```python
from build123d import *

# Parameters (mm, degrees)
F0_R     = 1.5
F0_W     = 8
F0_H     = 3.175
F0_W_2   = 31
F0_H_2   = 9
F0_W_3   = 12
F0_W_4   = 25
F1_DEPTH = 3.175


# Not quite as in the source:
# - a length typed as a fraction of an inch, garbled in the dataset ("3 / 203.2 mm" for 3/8 in), is restored
# - a feature names something its author has since deleted; it is built from what else it names


with BuildPart() as f1:
    # F0 (on Top) → F1 (new body)
    with BuildSketch(Plane.XY):
        Polygon((7.0042573512, 24.8119444549), (-17.9957426488, 24.8119444549), (-17.9957426488, 15.8119444549), (7.0042573512, 15.8119444549), (22.5042573512, 15.8119444549), (38.0042573512, 15.8119444549), (63.0042573512, 15.8119444549), (63.0042573512, 24.8119444549), (38.0042573512, 24.8119444549), align=None)
        with Locations((-13.4957426488, 20.3119444549)):
            Circle(F0_R, mode=Mode.SUBTRACT)
        with Locations((58.5042573512, 20.3119444549)):
            Circle(F0_R, mode=Mode.SUBTRACT)
        Polygon((7.0042573512, 40.6369444549), (7.0042573512, 24.8119444549), (38.0042573512, 24.8119444549), (38.0042573512, 40.6369444549), (30.0042573512, 40.6369444549), (24.0042573512, 40.6369444549), (24.0042573512, 31.3119444549), (25.5042573512, 31.3119444549), (25.5042573512, 29.3119444549), (24.0042573512, 29.3119444549), (24.0042573512, 27.8119444549), (21.0042573512, 27.8119444549), (21.0042573512, 29.3119444549), (19.5042573512, 29.3119444549), (19.5042573512, 31.3119444549), (21.0042573512, 31.3119444549), (21.0042573512, 40.6369444549), (15.0042573512, 40.6369444549), align=None)
        with Locations((11.0042573512, 42.2244444549)):
            Rectangle(F0_W, F0_H)
        Polygon((22.5042573512, 15.8119444549), (7.0042573512, 15.8119444549), (7.0042573512, -12.1880555451), (38.0042573512, -12.1880555451), (38.0042573512, 15.8119444549), align=None)
        with Locations((34.0042573512, 42.2244444549)):
            Rectangle(F0_W, F0_H)
        with Locations((22.5042573512, -16.6880555451)):
            Rectangle(F0_W_2, F0_H_2)
        with Locations((1.0042573512, -16.6880555451)):
            Rectangle(F0_W_3, F0_H_2)
        with Locations((-0.4957426488, -16.6880555451)):
            Circle(F0_R, mode=Mode.SUBTRACT)
        Polygon((38.0042573512, -21.1880555451), (7.0042573512, -21.1880555451), (7.0042573512, -29.0130555451), (15.0042573512, -29.0130555451), (21.0042573512, -29.0130555451), (21.0042573512, -25.6880555451), (19.5042573512, -25.6880555451), (19.5042573512, -23.6880555451), (21.0042573512, -23.6880555451), (21.0042573512, -22.1880555451), (24.0042573512, -22.1880555451), (24.0042573512, -23.6880555451), (25.5042573512, -23.6880555451), (25.5042573512, -25.6880555451), (24.0042573512, -25.6880555451), (24.0042573512, -29.0130555451), (30.0042573512, -29.0130555451), (38.0042573512, -29.0130555451), align=None)
        with Locations((50.5042573512, -16.6880555451)):
            Rectangle(F0_W_4, F0_H_2)
        with Locations((58.5042573512, -16.6880555451)):
            Circle(F0_R, mode=Mode.SUBTRACT)
        with Locations((11.0042573512, -30.6005555451)):
            Rectangle(F0_W, F0_H)
        with Locations((34.0042573512, -30.6005555451)):
            Rectangle(F0_W, F0_H)
    extrude(amount=F1_DEPTH)


solid = f1.part
```
Here's how the part is built. I have some questions about the finished solid (model axes, mm). A direction names the side the tool comes from. Round coordinates to 2 decimals unless told otherwise and drop trailing zeros. Order: outer loops, then holes, each group sorted by start corner. A loop starts at its lowest first (then second) coordinate and runs counter-clockwise, first axis right, second up. Notation, with made-up numbers: (32, 63) -> (43, 63) arc R29 cw to (43, 89) -> close; hole circle Ø11 at (77.5, 53.5). An arc over 180 degrees is marked (long way). Use a Markdown table: item, result. Add a question column.
(1) Suppose I cut it at B-B, the plane x = 58. Please give me the cut outline in (y, z) (3 decimals).
(2) For pin 1 Ø12 at (x, y) = (1.5, 3.5) entering from -Z; pin 2 Ø1 at (y, z) = (-31, 2.5) entering from -X; pin 3 Ø1.6 at (x, z) = (17, 1) entering from -Y; pin 4 Ø1.6 at (y, z) = (-23, 1.5) entering from +X, each with a flat end and sliding along its axis, tell me the tip position at first contact or that it passes through.
(3) Suppose I cut it at A-A, the plane y = 38.5. Please give me the cut outline in (x, z) (3 decimals), and give its area (3 significant figures).
(4) For faces 4 (the face through (7.004, 34, 2)), 5 (the face through (51, 24.812, 2)), 6 (the face through (15.004, 42, 2)), 7 (the face through (50, -12.188, 2)), 8 (the face through (25.504, -25, 2)), which set-ups out of +Z, -Z, +X, -X, +Y, -Y let a thin tool reach every point of the face, with its end or its side?
(5) Suppose I cut it at C-C, the plane y = -3. Please give me the cut outline in (x, z) (3 decimals), and give its area (3 significant figures).
(6) I need wall thicknesses on line 1 along Y through (x, z) = (20.5, 1.2); line 2 along Y through (x, z) = (54.5, 0.35); line 3 along X through (y, z) = (32.5, 0.3). Which ranges of each line are inside material? Lowest first, please.
(7) Suppose I cut it at D-D, the plane x = -11. Please give me the cut outline in (y, z) (3 decimals).
(8) If we mould it in two halves opening along Y, with no side actions, what happens to faces 1 (the face through (59.89, 19.74, 1.57)), 2 (the face through (38.004, -27, 2)), 3 (the face through (27, -29.013, 2))? For each: released by +Y, released by -Y, zero draft, split by the parting line, or undercut.
Verdict:
| question | item | result |
|---|---|---|
| 1 | outline | (-21.188, 0) -> (-18.101, 0) -> (-18.101, 3.175) -> (-21.188, 3.175) -> close; (-15.275, 0) -> (-12.188, 0) -> (-12.188, 3.175) -> (-15.275, 3.175) -> close; (15.812, 0) -> (18.899, 0) -> (18.899, 3.175) -> (15.812, 3.175) -> close; (21.725, 0) -> (24.812, 0) -> (24.812, 3.175) -> (21.725, 3.175) -> close |
| 2 | pin 1 | z = 0 |
| 2 | pin 2 | x = 7 |
| 2 | pin 3 | y = -29.01 |
| 2 | pin 4 | x = 38 |
| 3 | outline | (7.004, 0) -> (21.004, 0) -> (21.004, 3.175) -> (7.004, 3.175) -> close; (24.004, 0) -> (38.004, 0) -> (38.004, 3.175) -> (24.004, 3.175) -> close |
| 3 | area | 88.9 mm2 |
| 4 | face 4 | +Z, -Z, -X, +Y |
| 4 | face 5 | +Z, -Z, +X, +Y |
| 4 | face 6 | +Z, -Z, +Y |
| 4 | face 7 | +Z, -Z, +X |
| 4 | face 8 | +Z, -Z |
| 5 | outline | (7.004, 0) -> (38.004, 0) -> (38.004, 3.175) -> (7.004, 3.175) -> close |
| 5 | area | 98.4 mm2 |
| 6 | line 1 | -29.01 to -25.69, -23.69 to 29.31, 31.31 to 40.64 |
| 6 | line 2 | -21.19 to -12.19, 15.81 to 24.81 |
| 6 | line 3 | 7 to 21, 24 to 38 |
| 7 | outline | (15.812, 0) -> (24.812, 0) -> (24.812, 3.175) -> (15.812, 3.175) -> close |
| 8 | face 1 | undercut |
| 8 | face 2 | zero draft |
| 8 | face 3 | released by -Y |
